Part print with two shaded views. Sizes in mm from the minimum x, y, z corner. Coordinates: 2 decimals unless noted, no trailing zeros. Loops run counter-clockwise (first coordinate to the right, second up) from the corner with the lowest first, then second, coordinate; pieces in that order, holes last.
(1) Slice it at A-A (z = 52). Give the cut face in (x, y), and give its area (3 significant figures).
(2) Wall check: L1, parallel to Y at x = 12.7, z = 7.5; L2, parallel to Y at x = 12.7, z = 137.5. Give the ranges that are in metal, low to high.
(3) Flat gauge pins, fed straight in: P1, Ø10, axis at y = 12, z = 29, coming from the -X side; P2, Ø1.2, axis at x = 21, y = 13, coming from the -Z side; P3, Ø2, axis at y = 17.5, z = 94.5, coming from the +X side; P4, Ø5, axis at y = 21.5, z = 96.5, coming from the -X side. Where does each tip first touch, or does it go through?
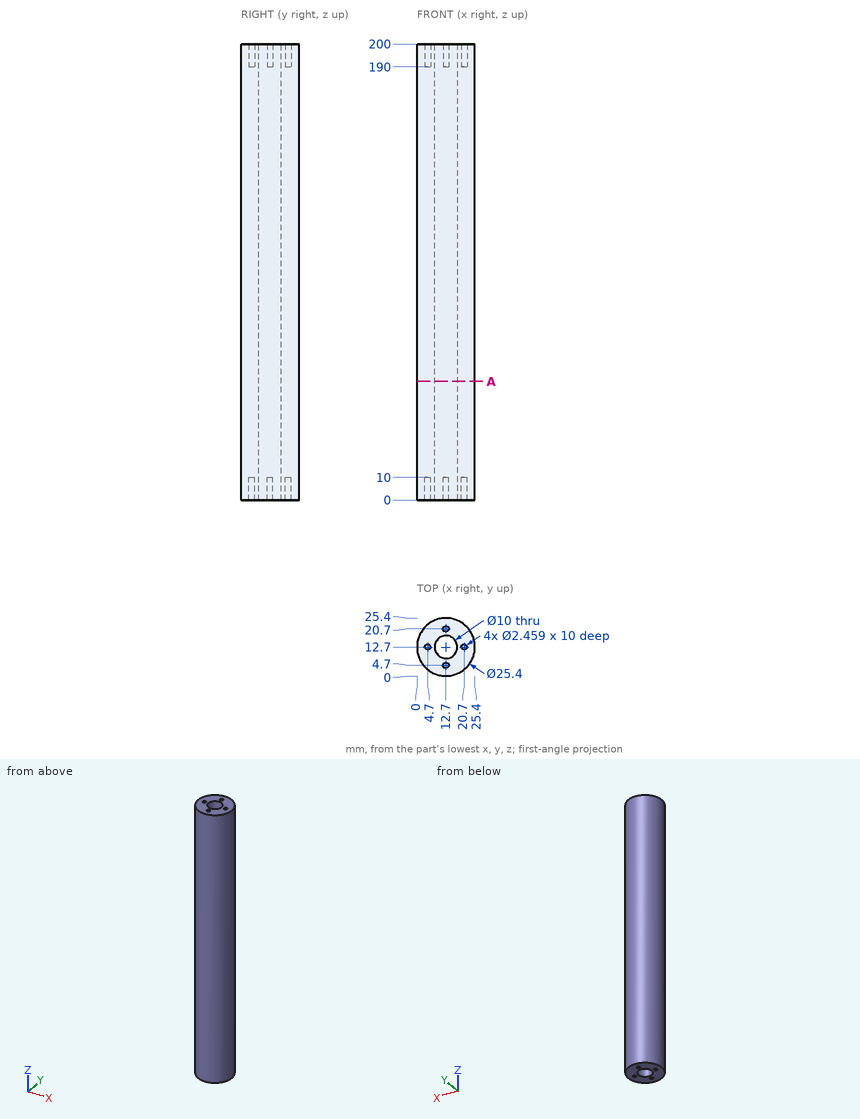
Response values:
1. outline: circle Ø25.4 at (12.7, 12.7); hole circle Ø10 at (12.7, 12.7)
1. area: 428 mm2
2. L1: y = 0 to 3.47, 5.93 to 7.7, 17.7 to 19.47, 21.93 to 25.4
2. L2: y = 0 to 7.7, 17.7 to 25.4
3. P1: stops at x = 0
3. P2: stops at z = 10
3. P3: stops at x = 24.82
3. P4: stops at x = 1.67
